```python
from build123d import *

# Parameters (mm, degrees)
F0_R     = 6.5
F1_DEPTH = 50
F2_R     = 5.334
F4_DEPTH = 40
F5_R     = 5.5
F6_DEPTH = 0.5


with BuildPart() as f1:
    # F0 (on Front) → F1 (new body)
    with BuildSketch(Plane.XZ):
        Circle(F0_R)
    extrude(amount=F1_DEPTH)

    # F2
    f2_edges = [f1.edges().sort_by_distance(p)[0] for p in [
        (-6.5, -50, 0),
    ]]
    fillet(f2_edges, radius=F2_R)

    # F3 (on face) → F4 (cut)
    with BuildSketch(Plane.XZ.offset(50)):
        with BuildLine():
            Line((-0.5, 1.0533546411), (-0.5, 4.9749371855))
            ThreePointArc((-0.5, 4.9749371855), (-3.5355339059, 3.5355339059), (-4.9749371855, 0.5))
            Line((-4.9749371855, 0.5), (-1.0533546411, 0.5))
            ThreePointArc((-1.0533546411, 0.5), (-0.8244865069, 0.8244865069), (-0.5, 1.0533546411))
        make_face()
        with BuildLine():
            Line((1.0533546411, 0.5), (4.9749371855, 0.5))
            ThreePointArc((4.9749371855, 0.5), (3.5355339059, 3.5355339059), (0.5, 4.9749371855))
            Line((0.5, 4.9749371855), (0.5, 1.0533546411))
            ThreePointArc((0.5, 1.0533546411), (0.8244865069, 0.8244865069), (1.0533546411, 0.5))
        make_face()
        with BuildLine():
            ThreePointArc((0.5, -4.9749371855), (3.5355339059, -3.5355339059), (4.9749371855, -0.5))
            Line((4.9749371855, -0.5), (1.0533546411, -0.5))
            ThreePointArc((1.0533546411, -0.5), (0.8244865069, -0.8244865069), (0.5, -1.0533546411))
            Line((0.5, -1.0533546411), (0.5, -4.9749371855))
        make_face()
        with BuildLine():
            ThreePointArc((-4.9749371855, -0.5), (-3.5355339059, -3.5355339059), (-0.5, -4.9749371855))
            Line((-0.5, -4.9749371855), (-0.5, -1.0533546411))
            ThreePointArc((-0.5, -1.0533546411), (-0.8244865069, -0.8244865069), (-1.0533546411, -0.5))
            Line((-1.0533546411, -0.5), (-4.9749371855, -0.5))
        make_face()
    extrude(amount=-F4_DEPTH, mode=Mode.SUBTRACT)

    # F5 (on face) → F6 (cut)
    with BuildSketch(Plane(origin=(0, 0, 0), x_dir=(-1, 0, 0), z_dir=(0, 1, 0))):
        Circle(F5_R)
    extrude(amount=-F6_DEPTH, mode=Mode.SUBTRACT)


solid = f1.part
```
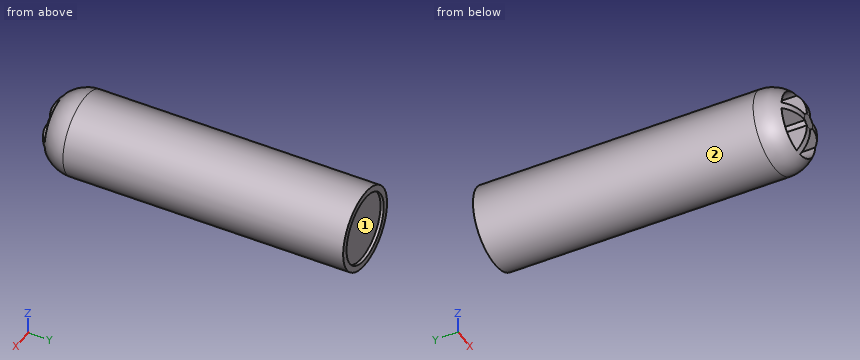
Could you check a few things on this model? Use its own coordinates, in mm. Face numbers are marked on the shaded views. Give positions to 0.01 mm unless a question says otherwise; leave off trailing zeros. Order: outer loops, then holes, each group sorted by start corner. A loop starts at its lowest first (then second) coordinate and runs counter-clockwise, first axis right, second up.
Q1. Suppose I cut it at A-A, the plane y = -26. Write out the boundary of the cut face in (x, z), and give its area (3 significant figures).
Q2. We'd pull the mould along Z, two halves only. Please class the marked faces 1 and 2: +Z half, -Z half, draft (parallel to the pull), parting line (faces both ways), or undercut.
Q3. If I drill on line 1 along X through (y, z) = (-24, 1.25); line 2 along X through (y, z) = (-40.5, -3); line 3 along Z through (x, y) = (1, -23), over which ranges is the centre line in solid material (lowest first)?
Q4. I'm going to push flat-ended pins straight in: P1, Ø1.3, axis at x = 4, z = 3, coming from the -Y side; P2, Ø1.2, axis at y = -39, z = -3, coming from the -X side; P3, Ø3.5, axis at x = -0.5, z = -2.5, coming from the +Y side. Where does each tip first touch, or does it pass through?
Q5. Suppose I cut it at B-B, the plane y = -6. Write out the boundary of the cut face in (x, z), and give its area (3 significant figures).
Solution:
1. outline: circle Ø13 at (0, 0); hole (-4.97, -0.5) arc R5 ccw to (-0.5, -4.97) - (-0.5, -1.05) arc R1.17 cw to (-1.05, -0.5) - close; hole (-4.97, 0.5) - (-1.05, 0.5) arc R1.17 cw to (-0.5, 1.05) - (-0.5, 4.97) arc R5 ccw to start; hole (0.5, -4.97) arc R5 ccw to (4.97, -0.5) - (1.05, -0.5) arc R1.17 cw to (0.5, -1.05) - close; hole (0.5, 1.05) arc R1.17 cw to (1.05, 0.5) - (4.97, 0.5) arc R5 ccw to (0.5, 4.97) - close
1. area: 73.9 mm2
2. face 1: undercut
2. face 2: parting line
3. line 1: x = -6.38 to -4.84, -0.5 to 0.5, 4.84 to 6.38
3. line 2: x = -5.77 to -4, -0.5 to 0.5, 4 to 5.77
3. line 3: z = -6.42 to -4.9, -0.6 to 0.6, 4.9 to 6.42
4. P1: stops at y = -48.37
4. P2: stops at x = -6.04
4. P3: stops at y = -0.5
5. outline: circle Ø13 at (0, 0)
5. area: 133 mm2
